Can you work these out from the model? Positions are in its coordinate system, mm. Face numbers are marked on the shaded views. A direction names the side the tool comes from. Round coordinates to 2 decimals unless told otherwise and drop trailing zeros. Order: outer loops, then holes, each group sorted by start corner. A loop starts at its lowest first (then second) coordinate and runs counter-clockwise, first axis right, second up. Notation, with made-up numbers: M 29,-9.5 L 87,-9.5 A11 ccw 87,7.5 Z; hole C 48,54 d10. An arc over 180 degrees is marked long. Answer as a JSON object with one key per item and string values. Group by question number.
```python
from build123d import *

# Parameters (mm, degrees)
BOX010_W     = 4
BOX010_H     = 1
BOX010_DEPTH = 1.3
BOX001_W     = 9
BOX001_H     = 12
BOX001_DEPTH = 4.6
FILLET_R     = 1


with BuildPart() as cube010:
    # Box010 → Box010 (new body)
    with BuildSketch(Plane(origin=(-2, -6.5, 5.1), x_dir=(1, 0, 0), z_dir=(0, 0, 1))):
        with Locations((2, 0.5)):
            Rectangle(BOX010_W, BOX010_H)
    extrude(amount=BOX010_DEPTH)


with BuildPart() as cut005:
    # Box001 → Box001 (new body)
    with BuildSketch(Plane(origin=(-4.5, -6.5, 1.8), x_dir=(1, 0, 0), z_dir=(0, 0, 1))):
        with Locations((4.5, 6)):
            Rectangle(BOX001_W, BOX001_H)
    extrude(amount=BOX001_DEPTH)

    # Fillet
    fillet_edges = [cut005.edges().sort_by_distance(p)[0] for p in [
        (-4.5, -6.5, 4.1),
        (-4.5, 5.5, 4.1),
        (4.5, -6.5, 4.1),
        (4.5, 5.5, 4.1),
    ]]
    fillet(fillet_edges, radius=FILLET_R)

    # Cut005: cut Cube010
    add(cube010.part, mode=Mode.SUBTRACT)


solid = cut005.part
```
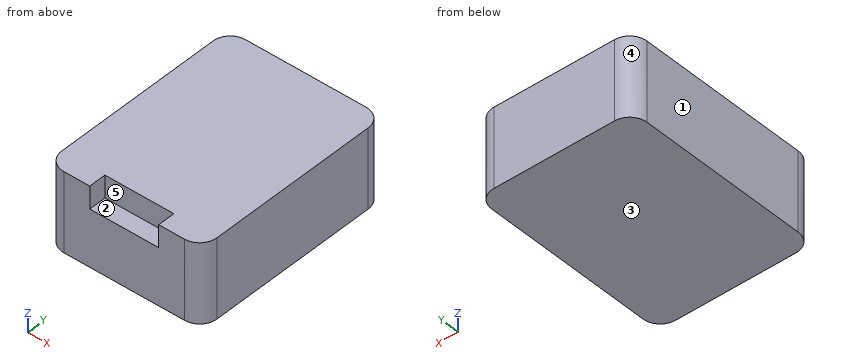
1) We'd pull the mould along X, two halves only. Please class the marked faces 3, 4 and 5: +X half, -X half, draft (parallel to the pull), parting line (faces both ways), or undercut.
2) For pin 1 (0.5 mm diameter, centred on y = -6, z = 6, fed in from +X); pin 2 (0.6 mm diameter, centred on x = -0.5, z = 5.5, fed in from -Y), each with a flat end and sliding along its axis, tell me the tip position at first contact or that it passes through.
3) If we section it at B-B on x = 0: Write out the boundary of the cut face in (y, z).
4) I need wall thicknesses on line 1 along Y through (x, z) = (-3.75, 3.9); line 2 along Y through (x, z) = (4.25, 3.9); line 3 along X through (y, z) = (5.25, 2.55). Which ranges of each line are inside material? Lowest first, please.
5) If we section it at A-A on z = 5.6: Write out the boundary of the cut face in (x, y).
6) Which directions (+Z, -Z, +X, -X, +Y, -Y) give clear straight access to the entire face, cutting with the end or side of a thin tool? Please do the marked faces 1 and 2.
Findings:
{
 "1": {"face 3": "draft", "face 4": "-X half", "face 5": "undercut"},
 "2": {"pin 1": "stops at x = 4.47", "pin 2": "stops at y = -5.5"},
 "3": {"outline": "M -6.5,1.8 L 5.5,1.8 L 5.5,6.4 L -5.5,6.4 L -5.5,5.1 L -6.5,5.1 Z"},
 "4": {"line 1": "y = -6.47 to 5.47", "line 2": "y = -6.16 to 5.16", "line 3": "x = -4.16 to 4.16"},
 "5": {"outline": "M -4.5,-5.5 A1 ccw -3.5,-6.5 L -2,-6.5 L -2,-5.5 L 2,-5.5 L 2,-6.5 L 3.5,-6.5 A1 ccw 4.5,-5.5 L 4.5,4.5 A1 ccw 3.5,5.5 L -3.5,5.5 A1 ccw -4.5,4.5 Z"},
 "6": {"face 1": "+Z, -Z, -X, +Y, -Y", "face 2": "+Z, -Y"}
}
